Here's how the part is built. I have some questions about the finished solid (model axes, mm). Coordinates: 2 decimals unless noted, no trailing zeros. Order: outer loops, then holes, each group sorted by start corner. A loop starts at its lowest first (then second) coordinate and runs counter-clockwise, first axis right, second up. Notation, with made-up numbers: M 49.5,82 L 74.5,82 A22 cw 74.5,116 Z; hole C 57,56.5 d8. An arc over 180 degrees is marked long. Answer as CSV lines item,"result". Start each with the question number.
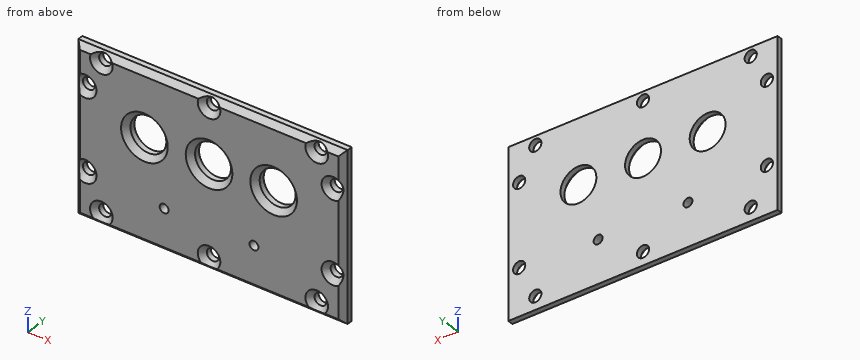
```python
from build123d import *

# Parameters (mm, degrees)
SKETCH_1_W                 = 75
SKETCH_1_H                 = 47
SKETCH_1_R                 = 5
EXTRUDE_731_DEPTH          = 3
HOLE_WIZARD_M3_AT_2_COUNT  = 2
HOLE_WIZARD_M3_AT_2_PITCH  = 30
HOLE_WIZARD_M3_AT_3_COUNT  = 2
HOLE_WIZARD_M3_AT_3_PITCH  = 30
HOLE_WIZARD_M3_AT_4_COUNT  = 2
HOLE_WIZARD_M3_AT_4_PITCH  = 40.75
HOLE_WIZARD_M3_AT_5_COUNT  = 2
HOLE_WIZARD_M3_AT_5_PITCH  = 50.602000949
HOLE_WIZARD_M3_AT_6_COUNT  = 2
HOLE_WIZARD_M3_AT_6_PITCH  = 50.602000949
HOLE_WIZARD_M3_AT_7_COUNT  = 2
HOLE_WIZARD_M3_AT_7_PITCH  = 35.472700771
HOLE_WIZARD_M3_AT_8_COUNT  = 2
HOLE_WIZARD_M3_AT_8_PITCH  = 35.472700771
HOLE_WIZARD_M3_AT_9_COUNT  = 2
HOLE_WIZARD_M3_AT_9_PITCH  = 46.549033287
HOLE_WIZARD_M3_AT_10_COUNT = 2
HOLE_WIZARD_M3_AT_10_PITCH = 46.549033287
HOLE_WIZARD_M3_2_D         = 2.5
CHAMFER_1_SIZE             = 1.5


with BuildPart() as part:
    # Эскиз1 → Extrude 731 (new body)
    with BuildSketch(Plane(origin=(0, 0, 0), x_dir=(1, 0, 0), z_dir=(0, 1, 0))):
        with Locations((0, -23.5)):
            Rectangle(SKETCH_1_W, SKETCH_1_H)
        with Locations(Location((18, -29, 0), (0, 0, 270))):
            Circle(SKETCH_1_R, mode=Mode.SUBTRACT)
        with Locations(Location((-18, -29, 0), (0, 0, 270))):
            Circle(SKETCH_1_R, mode=Mode.SUBTRACT)
        with Locations(Location((0, -29, 0), (0, 0, 270))):
            Circle(SKETCH_1_R, mode=Mode.SUBTRACT)
    extrude(amount=EXTRUDE_731_DEPTH)

    # Эскиз3 → Hole Wizard M3 (revolve, cut)
    with BuildSketch(Plane(origin=(0, 0, 44.5), x_dir=(0, 0, -1), z_dir=(1, 0, 0))):
        Polygon((0, 0), (0, 3), (1.7, 3), (1.7, 1.45), (3.15, 0), align=None)
    hole_wizard_m3 = revolve(axis=Axis((0, -6.35, 44.5), (0, 1, 0)), mode=Mode.SUBTRACT)

    # Hole Wizard M3 at 2: Hole Wizard M3 ×2
    with Locations(*[(i * HOLE_WIZARD_M3_AT_2_PITCH, 0, 0) for i in range(1, HOLE_WIZARD_M3_AT_2_COUNT)]):
        add(hole_wizard_m3, mode=Mode.SUBTRACT)

    # Hole Wizard M3 at 3: Hole Wizard M3 ×2
    with Locations(*[(-i * HOLE_WIZARD_M3_AT_3_PITCH, 0, 0) for i in range(1, HOLE_WIZARD_M3_AT_3_COUNT)]):
        add(hole_wizard_m3, mode=Mode.SUBTRACT)

    # Hole Wizard M3 at 4: Hole Wizard M3 ×2
    with Locations(*[(0, 0, -i * HOLE_WIZARD_M3_AT_4_PITCH) for i in range(1, HOLE_WIZARD_M3_AT_4_COUNT)]):
        add(hole_wizard_m3, mode=Mode.SUBTRACT)

    # Hole Wizard M3 at 5: Hole Wizard M3 ×2
    with Locations(*[Vector(-0.5928619311020034, 0, -0.8053041230802209) * (i * HOLE_WIZARD_M3_AT_5_PITCH) for i in range(1, HOLE_WIZARD_M3_AT_5_COUNT)]):
        add(hole_wizard_m3, mode=Mode.SUBTRACT)

    # Hole Wizard M3 at 6: Hole Wizard M3 ×2
    with Locations(*[Vector(0.5928619311020034, 0, -0.8053041230802209) * (i * HOLE_WIZARD_M3_AT_6_PITCH) for i in range(1, HOLE_WIZARD_M3_AT_6_COUNT)]):
        add(hole_wizard_m3, mode=Mode.SUBTRACT)

    # Hole Wizard M3 at 7: Hole Wizard M3 ×2
    with Locations(*[Vector(-0.972578891654415, 0, -0.23257321322170757) * (i * HOLE_WIZARD_M3_AT_7_PITCH) for i in range(1, HOLE_WIZARD_M3_AT_7_COUNT)]):
        add(hole_wizard_m3, mode=Mode.SUBTRACT)

    # Hole Wizard M3 at 8: Hole Wizard M3 ×2
    with Locations(*[Vector(0.972578891654415, 0, -0.23257321322170757) * (i * HOLE_WIZARD_M3_AT_8_PITCH) for i in range(1, HOLE_WIZARD_M3_AT_8_COUNT)]):
        add(hole_wizard_m3, mode=Mode.SUBTRACT)

    # Hole Wizard M3 at 9: Hole Wizard M3 ×2
    with Locations(*[Vector(0.7411539523694183, 0, -0.6713351017838932) * (i * HOLE_WIZARD_M3_AT_9_PITCH) for i in range(1, HOLE_WIZARD_M3_AT_9_COUNT)]):
        add(hole_wizard_m3, mode=Mode.SUBTRACT)

    # Hole Wizard M3 at 10: Hole Wizard M3 ×2
    with Locations(*[Vector(-0.7411539523694182, 0, -0.6713351017838932) * (i * HOLE_WIZARD_M3_AT_10_PITCH) for i in range(1, HOLE_WIZARD_M3_AT_10_COUNT)]):
        add(hole_wizard_m3, mode=Mode.SUBTRACT)

    # Hole Wizard M3 2 (through all)
    with Locations(Plane(origin=(0, 0, 0), x_dir=(-1, 0, 0), z_dir=(0, -1, 0))):
        with Locations((12.5, -12), (-12.5, -12)):
            Hole(HOLE_WIZARD_M3_2_D / 2)

    # Фаска1
    # the kernel refuses this chamfer: 1.5 mm, written as the material it takes off along each edge
    with BuildSketch(Plane(origin=(31.941147692, 0, 47), x_dir=(0, -0.02749587661058636, -0.9996219169112968), z_dir=(-1, 0, 0)), Plane(origin=(1.941147692, 0, 47), x_dir=(0, -0.02749587661058636, -0.9996219169112968), z_dir=(-1, 0, 0))) as chamfer_1_piece_1:
        Polygon((CHAMFER_1_SIZE * 0.999621916911, -CHAMFER_1_SIZE * 0.0274958766106), (-CHAMFER_1_SIZE * 0.0274958766106, -CHAMFER_1_SIZE * 0.999621916911), (0, 0), align=None)
    extrude(amount=33.882295385, mode=Mode.SUBTRACT)
    with BuildSketch(Plane(origin=(0, 0, 29), x_dir=(0, 0, 1), z_dir=(-1, 0, 0))) as chamfer_1_piece_2:
        Polygon((5 + CHAMFER_1_SIZE, 0), (5, CHAMFER_1_SIZE), (5, 0), align=None)
    revolve(axis=Axis((0, 0, 29), (0, 1, 0)), mode=Mode.SUBTRACT)
    with BuildSketch(Plane(origin=(18, 0, 29), x_dir=(0, 0, 1), z_dir=(-1, 0, 0))) as chamfer_1_piece_3:
        Polygon((5 + CHAMFER_1_SIZE, 0), (5, CHAMFER_1_SIZE), (5, 0), align=None)
    revolve(axis=Axis((18, 0, 29), (0, 1, 0)), mode=Mode.SUBTRACT)
    with BuildSketch(Plane(origin=(-18, 0, 29), x_dir=(0, 0, 1), z_dir=(-1, 0, 0))) as chamfer_1_piece_4:
        Polygon((5 + CHAMFER_1_SIZE, 0), (5, CHAMFER_1_SIZE), (5, 0), align=None)
    revolve(axis=Axis((-18, 0, 29), (0, 1, 0)), mode=Mode.SUBTRACT)
    with BuildSketch(Plane(origin=(-37.5, 0, 39.147055846), x_dir=(-0.027495876610586778, 0.9996219169112968, 0), z_dir=(0, 0, -1)), Plane(origin=(37.5, 0, 10.352944154), x_dir=(0.027495876610586778, 0.9996219169112968, 0), z_dir=(0, 0, 1))) as chamfer_1_piece_5:
        Polygon((CHAMFER_1_SIZE * 0.999621916911, CHAMFER_1_SIZE * 0.0274958766106), (-CHAMFER_1_SIZE * 0.0274958766106, CHAMFER_1_SIZE * 0.999621916911), (0, 0), align=None)
    extrude(amount=28.794111693, mode=Mode.SUBTRACT)
    with BuildSketch(Plane(origin=(37.5, 0, -3.857524482), x_dir=(0.027495876610586778, 0.9996219169112968, 0), z_dir=(0, 0, 1)), Plane(origin=(-37.5, 0, 16.147055846), x_dir=(-0.027495876610586778, 0.9996219169112968, 0), z_dir=(0, 0, -1))) as chamfer_1_piece_6:
        Polygon((CHAMFER_1_SIZE * 0.999621916911, CHAMFER_1_SIZE * 0.0274958766106), (-CHAMFER_1_SIZE * 0.0274958766106, CHAMFER_1_SIZE * 0.999621916911), (0, 0), align=None)
    extrude(amount=20.004580328, mode=Mode.SUBTRACT)
    with BuildSketch(Plane(origin=(-28.058852308, 0, 47), x_dir=(0, -0.02749587661058636, -0.9996219169112968), z_dir=(-1, 0, 0)), Plane(origin=(41.357524482, 0, 47), x_dir=(0, -0.02749587661058636, -0.9996219169112968), z_dir=(-1, 0, 0))) as chamfer_1_piece_7:
        Polygon((CHAMFER_1_SIZE * 0.999621916911, -CHAMFER_1_SIZE * 0.0274958766106), (-CHAMFER_1_SIZE * 0.0274958766106, -CHAMFER_1_SIZE * 0.999621916911), (0, 0), align=None)
    extrude(amount=13.298672174, mode=Mode.SUBTRACT)
    with BuildSketch(Plane(origin=(-41.357524482, 0, 0), x_dir=(0, 0.9996219169112968, -0.027495876610586372), z_dir=(1, 0, 0))) as chamfer_1_piece_8:
        Polygon((CHAMFER_1_SIZE * 0.999621916911, CHAMFER_1_SIZE * 0.0274958766106), (-CHAMFER_1_SIZE * 0.0274958766106, CHAMFER_1_SIZE * 0.999621916911), (0, 0), align=None)
    extrude(amount=82.715048964, mode=Mode.SUBTRACT)
    with BuildSketch(Plane(origin=(37.5, 0, 33.352944154), x_dir=(0.027495876610586778, 0.9996219169112968, 0), z_dir=(0, 0, 1)), Plane(origin=(-37.5, 0, 50.857524482), x_dir=(-0.027495876610586778, 0.9996219169112968, 0), z_dir=(0, 0, -1))) as chamfer_1_piece_9:
        Polygon((CHAMFER_1_SIZE * 0.999621916911, CHAMFER_1_SIZE * 0.0274958766106), (-CHAMFER_1_SIZE * 0.0274958766106, CHAMFER_1_SIZE * 0.999621916911), (0, 0), align=None)
    extrude(amount=17.504580328, mode=Mode.SUBTRACT)


solid = part.part
```
1) Will these pins go through, and if not, where does the flat tip stop? pin 1 Ø3 at (x, z) = (0, 44.5) entering from +Y; pin 2 Ø4.5 at (x, z) = (-34.5, 36.25) entering from -Y; pin 3 Ø4 at (x, z) = (-34.5, 13.25) entering from +Y; pin 4 Ø4 at (x, z) = (30, 44.5) entering from -Y.
2) Suppose I cut it at A-A on y = 2.3. Give the number of separate pieces and of enclosed holes in the cut face, plus the area to 3 significant figures.
3) Suppose I cut it at D-D on z = 36.25. Please give me the cut outline in (x, y) (3 decimals), plus the area to 3 significant figures.
4) Suppose I cut it at C-C on x = -8. Please give me the cut outline in (y, z), plus the area to 3 significant figures.
5) I need wall thicknesses on line 1 (X direction, y = 2.5, z = 36.25); line 2 (X direction, y = 2.05, z = 29); line 3 (X direction, y = 1.9, z = 44.5). Which ranges of each line are inside material? Lowest first, please. Write a range as [from, to].
6) Suppose I cut it at B-B on z = 29. Please give me the cut outline in (x, y).
Output:
1,pin 1,"through"
1,pin 2,"y = 0.9"
1,pin 3,"y = 3"
1,pin 4,"y = 1.15"
2,separate pieces,"1"
2,enclosed holes,"15"
2,area,"3,190 mm²"
3,outline,"M -37.5,1.5 L -36.825,0.825 L -36.2,1.45 L -36.2,3 L -37.5,3 Z; M -32.8,1.45 L -31.35,0 L 31.35,0 L 32.8,1.45 L 32.8,3 L -32.8,3 Z; M 36.2,1.45 L 36.825,0.825 L 37.5,1.5 L 37.5,3 L 36.2,3 Z"
3,area,"200 mm²"
4,outline,"M 0,1.5 L 1.5,0 L 3,0 L 3,47 L 1.5,47 L 0,45.5 Z"
4,area,"139 mm²"
5,line 1,"[-37.5, -36.2], [-32.8, 32.8], [36.2, 37.5]"
5,line 2,"[-37.5, -23], [-13, -5], [5, 13], [23, 37.5]"
5,line 3,"[-37.5, -31.7], [-28.3, -1.7], [1.7, 28.3], [31.7, 37.5]"
6,outline,"M -37.5,1.5 L -36,0 L -24.5,0 L -23,1.5 L -23,3 L -37.5,3 Z; M -13,1.5 L -11.5,0 L -6.5,0 L -5,1.5 L -5,3 L -13,3 Z; M 5,1.5 L 6.5,0 L 11.5,0 L 13,1.5 L 13,3 L 5,3 Z; M 23,1.5 L 24.5,0 L 36,0 L 37.5,1.5 L 37.5,3 L 23,3 Z"
